```python
from build123d import *

# Parameters (mm, degrees)
SKETCH_2_W          = 10.95
SKETCH_2_H          = 11.9
EXTRUDE_2_DEPTH     = 4
SKETCH_1_W          = 8.95
SKETCH_1_H          = 10.9
CUT_EXTRUDE_1_DEPTH = 3


with BuildPart() as part:
    # 草圖2 → 填料-伸長2 (new body)
    with BuildSketch(Plane.XY):
        with Locations((0, -0.5)):
            Rectangle(SKETCH_2_W, SKETCH_2_H)
    extrude(amount=EXTRUDE_2_DEPTH)

    # 草圖1 → 除料-伸長1 (cut)
    with BuildSketch(Plane.XY):
        Rectangle(SKETCH_1_W, SKETCH_1_H)
    extrude(amount=CUT_EXTRUDE_1_DEPTH, mode=Mode.SUBTRACT)


solid = part.part
```
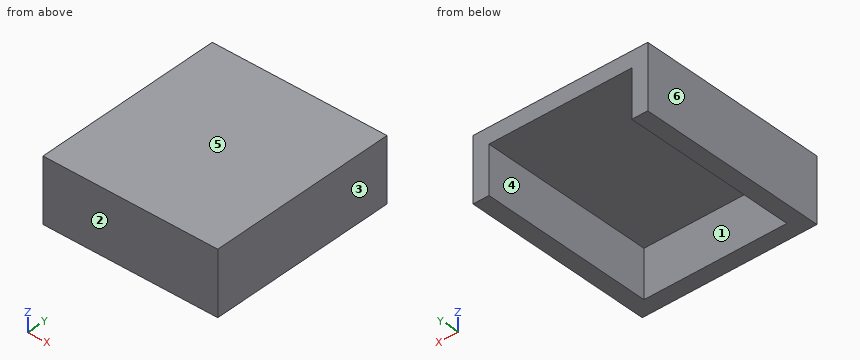
Here's how the part is built. I have some questions about the finished solid (model axes, mm). Face numbers are marked on the shaded views. A direction names the side the tool comes from. Coordinates: 2 decimals unless noted, no trailing zeros. Write each loop counter-clockwise with the first axis right and the second up, starting at its lowest first coordinate (ties: lowest second). Pieces come first, ordered by that corner, then holes. Notation, with made-up numbers: (-16, -33.75) -> (4, -33.75) arc R31 cw to (4, -1.75) -> close; hole circle Ø7 at (58, 27). An arc over 180 degrees is marked (long way). Use a Markdown table: item, result. Add a question column.
(1) I'm going to push flat-ended pins straight in: P1, Ø0.9, axis at x = 0.5, z = 2, coming from the +Y side; P2, Ø2.5, axis at x = 1, y = -1.5, coming from the -Z side. Where does each tip first touch, or does it pass through?
(2) If we section it at B-B, the plane y = 4.5: Write out the boundary of the cut face in (x, z) (3 decimals).
(3) If we section it at C-C, the plane z = 1.95: Write out the boundary of the cut face in (x, y) (3 decimals).
(4) For the marked faces 1 and 2, which set-ups out of +Z, -Z, +X, -X, +Y, -Y let a thin tool reach every point of the face, with its end or its side?
(5) If we section it at A-A, the plane x = -2.75: Write out the boundary of the cut face in (y, z), and give its area (3 significant figures).
(6) Please list where these lines run through material, in increasing order: line 1 (X direction, y = 1.5, z = 1.85) (3 decimals); line 2 (Z direction, x = -2, y = -2.75); line 3 (Y direction, x = 0, z = 2.6).
(7) We'd pull the mould along X, two halves only. Please class the marked faces 3, 4, 5 and 6: +X half, -X half, draft (parallel to the pull), parting line (faces both ways), or undercut.
Outcome:
| question | item | result |
|---|---|---|
| 1 | P1 | stops at y = -5.45 |
| 1 | P2 | stops at z = 3 |
| 2 | outline | (-5.475, 0) -> (-4.475, 0) -> (-4.475, 3) -> (4.475, 3) -> (4.475, 0) -> (5.475, 0) -> (5.475, 4) -> (-5.475, 4) -> close |
| 3 | outline | (-5.475, -6.45) -> (5.475, -6.45) -> (5.475, 5.45) -> (4.475, 5.45) -> (4.475, -5.45) -> (-4.475, -5.45) -> (-4.475, 5.45) -> (-5.475, 5.45) -> close |
| 4 | face 1 | -Z, +Y |
| 4 | face 2 | +Z, -Z, +X, -X, -Y |
| 5 | outline | (-6.45, 0) -> (-5.45, 0) -> (-5.45, 3) -> (5.45, 3) -> (5.45, 4) -> (-6.45, 4) -> close |
| 5 | area | 14.9 mm^2 |
| 6 | line 1 | x = -5.475 to -4.475, 4.475 to 5.475 |
| 6 | line 2 | z = 3 to 4 |
| 6 | line 3 | y = -6.45 to -5.45 |
| 7 | face 3 | +X half |
| 7 | face 4 | undercut |
| 7 | face 5 | draft |
| 7 | face 6 | -X half |
